Geometry: final body of the model. Coordinates: model frame, mm. Round coordinates to 2 decimals unless told otherwise and drop trailing zeros. Write each loop counter-clockwise with the first axis right and the second up, starting at its lowest first coordinate (ties: lowest second). Pieces come first, ordered by that corner, then holes. Notation, with made-up numbers: (84.25, -3.75) - (131.25, -3.75) arc R32 ccw to (131.25, 35.25) - close; hole circle Ø2 at (-10.5, -9.5). An arc over 180 degrees is marked (long way). Write each question's results on one line, items separated by ' | '.
Autodesk Inventor part; units mm, degrees
ref_plane "YZ Plane" through (0, 0, 0) normal (1, 0, 0) x (0, 1, 0)
ref_plane "XZ Plane" through (0, 0, 0) normal (0, 1, 0) x (-1, 0, 0)
ref_plane "XY Plane" through (0, 0, 0) normal (0, 0, 1) x (1, 0, 0)
sketch "Sketch1" plane through (0, 0, 0) normal (0, 1, 0) x (-1, 0, 0)
  line L0 (0.0672, -6.0996) -> (-626.6479, -12.9992)
  line L1 (0.0672, 6.0996) -> (-626.6479, 12.9992)
  arc A0 (0.0672, -6.0996) -> (0.0672, 6.0996) centre (0, 0) ccw
  arc A1 (-626.6479, 12.9992) -> (-626.6479, -12.9992) centre (-626.791, 0) ccw
  line L2 (-626.6327, 14.3791) -> (0.0823, 7.4795)
  arc A2 (0.0823, -7.4795) -> (0.0823, 7.4795) centre (0, 0) ccw
  line L3 (0.0823, -7.4795) -> (-626.6327, -14.3791)
  arc A3 (-626.6327, 14.3791) -> (-626.6327, -14.3791) centre (-626.791, 0) ccw
  dimension "d2" = 6.1
  dimension "d3" = 13
  dimension "d4" = 1.38
  dimension "d5" = 626.791
extrude "Extrusion1" add sketch "Sketch1" along normal blind 6
chamfer "Chamfer1" distance 0.2 angle 45 16 edges at (313.2904, 6, 9.5494) (-6.1, 6, 0) (313.2904, 6, -9.5494) (639.791, 6, 0) (313.2752, 6, 10.9293) (641.171, 6, 0) (313.2752, 6, -10.9293) (-7.48, 6, 0) (313.2752, 0, 10.9293) (-7.48, 0, 0) (313.2752, 0, -10.9293) (641.171, 0, 0) (313.2904, 0, 9.5494) (639.791, 0, 0) (313.2904, 0, -9.5494) (-6.1, 0, 0)
properties part number "x_axis_belt" material "Rubber"
Q1. Section query A-A, the plane z = 0. Return loops of the section in (x, y), plus the area to 3 significant figures.
Answer block:
outline: (-7.48, 0.2) - (-7.28, 0) - (-6.3, 0) - (-6.1, 0.2) - (-6.1, 5.8) - (-6.3, 6) - (-7.28, 6) - (-7.48, 5.8) - close; (639.79, 0.2) - (639.99, 0) - (640.97, 0) - (641.17, 0.2) - (641.17, 5.8) - (640.97, 6) - (639.99, 6) - (639.79, 5.8) - close | area: 16.4 mm2
Q2. Pin query (flat end, axial travel): pin 1 (3 mm diameter, centred on y = 4, z = 2.5, fed in from +X); pin 2 (3 mm diameter, centred on x = 540, y = 5, fed in from +Z); pin 3 (3 mm diameter, centred on x = 163.5, y = 5, fed in from -Z). Return the tip coordinate at first contact, or that it passes through.
Answer block:
pin 1: x = 641.14 | pin 2: z = 13.44 | pin 3: z = -9.3
Q3. Section query C-C, the plane x = 350. Return loops of the section in (y, z).
Answer block:
outline: (0, -11.13) - (0.2, -11.33) - (5.8, -11.33) - (6, -11.13) - (6, -10.15) - (5.8, -9.95) - (0.2, -9.95) - (0, -10.15) - close; (0, 10.15) - (0.2, 9.95) - (5.8, 9.95) - (6, 10.15) - (6, 11.13) - (5.8, 11.33) - (0.2, 11.33) - (0, 11.13) - close
Q4. Section query B-B, the plane y = 4.25. Return loops of the section in (x, z).
Answer block:
outline: (-0.08, -7.48) - (626.63, -14.38) arc R14.38 ccw (long way) to (626.63, 14.38) - (-0.08, 7.48) arc R7.48 ccw to start; hole (-0.07, -6.1) - (626.65, -13) arc R13 ccw (long way) to (626.65, 13) - (-0.07, 6.1) arc R6.1 ccw to start
Q5. Mould query, pull axis X, two halves, no side actions, for faces 1 (the cylindrical face through (639.788, 2.961, -0.288)), 2 (the flat face through (318, 6, -10)). Classes: pulls with the +X half, pulls with the -X half, needs draft (parallel to the pull), parting line crosses it, or undercut.
Answer block:
face 1: undercut | face 2: needs draft
Q6. Ray query, line 1 along Z through (x, y) = (343, 2.5); line 2 along Z through (x, y) = (295.5, 2); line 3 along X through (y, z) = (0.5, 4.75). Return the intervals inside material, ascending.
Answer block:
line 1: -11.26 to -9.88, 9.88 to 11.26 | line 2: -10.73 to -9.35, 9.35 to 10.73 | line 3: -5.78 to -3.83, 638.89 to 640.36
